from build123d import *

# Parameters (mm, degrees)
SKETCH_3_R          = 1.85
CUT_EXTRUDE_1_DEPTH = 20
SKETCH_4_R          = 1.85
CUT_EXTRUDE_2_DEPTH = 20


with BuildPart() as part:
    # Эскиз1 → По сечениям1 section 0
    with BuildSketch(Plane(origin=(0, 0, 0), x_dir=(1, 0, 0), z_dir=(0, 1, 0))):
        with BuildLine():
            Line((-66.449008168, -45.061574365), (66.449008168, -45.061574365))
            Line((66.449008168, -45.061574365), (66.449008168, 45.061574365))
            Line((66.449008168, 45.061574365), (-66.449008168, 45.061574365))
            Line((-66.449008168, 45.061574365), (-66.449008168, -45.061574365))
        make_face()
    # Эскиз2 → По сечениям1 section 1
    with BuildSketch(Plane(origin=(0, 10, 0), x_dir=(1, 0, 0), z_dir=(0, 1, 0))):
        with BuildLine():
            Line((56.449008168, 35.061574365), (-56.449008168, 35.061574365))
            Line((-56.449008168, 35.061574365), (-56.449008168, -35.061574365))
            Line((-56.449008168, -35.061574365), (56.449008168, -35.061574365))
            Line((56.449008168, -35.061574365), (56.449008168, 35.061574365))
        make_face()
    loft()

    # Эскиз3 → Вырез-Вытянуть1 (cut)
    with BuildSketch(Plane.XY.offset(45.061574365)):
        with Locations((51.449008168, 5)):
            Circle(SKETCH_3_R)
        with Locations(Location((-51.449008168, 5, 0), (0, 0, 270))):
            Circle(SKETCH_3_R)
    cut_extrude_1 = extrude(amount=-CUT_EXTRUDE_1_DEPTH, mode=Mode.SUBTRACT)

    # Зеркальное отражение1: Вырез-Вытянуть1 across plane
    add(cut_extrude_1.mirror(Plane.XY), mode=Mode.SUBTRACT)

    # Эскиз4 → Вырез-Вытянуть2 (cut)
    with BuildSketch(Plane(origin=(66.449008168, 0, 0), x_dir=(0, 0, -1), z_dir=(1, 0, 0))):
        with Locations((-20.061574365, 5)):
            Circle(SKETCH_4_R)
        with Locations(Location((20.061574365, 5, 0), (0, 0, 270))):
            Circle(SKETCH_4_R)
    cut_extrude_2 = extrude(amount=-CUT_EXTRUDE_2_DEPTH, mode=Mode.SUBTRACT)

    # Зеркальное отражение2: Вырез-Вытянуть2 across plane
    add(cut_extrude_2.mirror(Plane(origin=(0, 0, 0), x_dir=(0, 0, 1), z_dir=(1, 0, 0))), mode=Mode.SUBTRACT)


solid = part.part
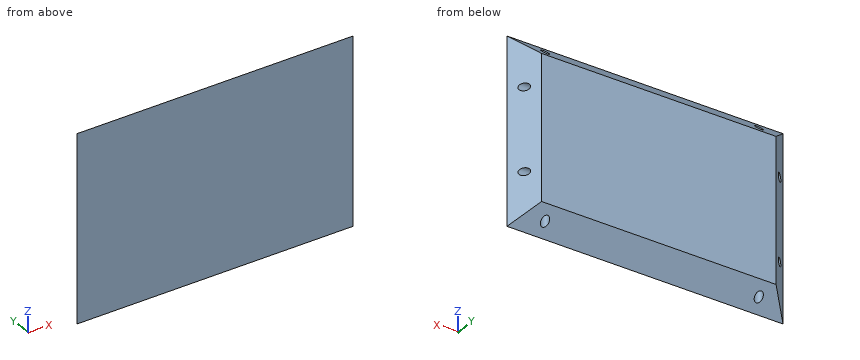
The listing builds one solid part. Answer for the finished solid, in the listing's coordinates (mm). Coordinates: 2 decimals unless noted, no trailing zeros. Answer in a Markdown table with one row per item. Add a question column.
Item 1: Each of these flat-tipped pins is pushed along its axis until it touches: P1, Ø6, axis at y = 5, z = 20.06, coming from the +X side; P2, Ø1, axis at x = 37, z = 36, coming from the +Y side; P3, Ø3.5, axis at x = -51.45, y = 5, coming from the -Z side. Where does it stop, or does it pass through?
Item 2: Find section A-A (z = -32.5). State how many separate pieces and enclosed holes the cut face has, then the cut area to 3 significant figures.
Item 3: Find the intervals of material crossed by L1, parallel to Z at x = -52, y = 5; L2, parallel to Z at x = 56.5, y = 5; L3, parallel to X at y = 5, z = 37.75, in increasing order. Write a range as from..to.
Result set:
| question | item | result |
|---|---|---|
| 1 | P1 | stops at x = 64.45 |
| 1 | P2 | stops at y = 9.56 |
| 1 | P3 | stops at z = -25.06 |
| 2 | separate pieces | 1 |
| 2 | enclosed holes | 2 |
| 2 | area | 1,210 mm² |
| 3 | L1 | z = -25.06..-21.91, -18.21..18.21, 21.91..25.06 |
| 3 | L2 | z = -40.06..-21.91, -18.21..18.21, 21.91..40.06 |
| 3 | L3 | x = -61.45..-53.3, -49.6..49.6, 53.3..61.45 |
